from build123d import *

# Parameters (mm, degrees)
SKETCH_1_W      = 18
SKETCH_1_H      = 3
SKETCH_1_R      = 1.6
EXTRUDE_1_DEPTH = 1
FILLET_1_R      = 3
FILLET_2_R      = 1


with BuildPart() as part:
    # 草图1 → 凸台-拉伸1 (new body)
    with BuildSketch(Plane(origin=(0, 0, 0), x_dir=(1, 0, 0), z_dir=(0, 1, 0))):
        with BuildLine():
            Line((21, 20), (-21, 20))
            Line((-21, 20), (-34.150684932, 4.931506849))
            ThreePointArc((-34.150684932, 4.931506849), (-36, 0), (-34.150684932, -4.931506849))
            Line((-34.150684932, -4.931506849), (-21, -20))
            Line((-21, -20), (21, -20))
            Line((21, -20), (34.150684932, -4.931506849))
            ThreePointArc((34.150684932, -4.931506849), (36, 0), (34.150684932, 4.931506849))
            Line((34.150684932, 4.931506849), (21, 20))
        make_face()
        with Locations((-12, -15)):
            Rectangle(SKETCH_1_W, SKETCH_1_H, mode=Mode.SUBTRACT)
        with Locations((-12, -9)):
            Rectangle(SKETCH_1_W, SKETCH_1_H, mode=Mode.SUBTRACT)
        with Locations((-12, -3)):
            Rectangle(SKETCH_1_W, SKETCH_1_H, mode=Mode.SUBTRACT)
        with Locations((12, -15)):
            Rectangle(SKETCH_1_W, SKETCH_1_H, mode=Mode.SUBTRACT)
        with Locations((12, -9)):
            Rectangle(SKETCH_1_W, SKETCH_1_H, mode=Mode.SUBTRACT)
        with Locations((12, -3)):
            Rectangle(SKETCH_1_W, SKETCH_1_H, mode=Mode.SUBTRACT)
        with Locations((-12, 3)):
            Rectangle(SKETCH_1_W, SKETCH_1_H, mode=Mode.SUBTRACT)
        with Locations((-12, 9)):
            Rectangle(SKETCH_1_W, SKETCH_1_H, mode=Mode.SUBTRACT)
        with Locations((-12, 15)):
            Rectangle(SKETCH_1_W, SKETCH_1_H, mode=Mode.SUBTRACT)
        with Locations((12, 3)):
            Rectangle(SKETCH_1_W, SKETCH_1_H, mode=Mode.SUBTRACT)
        with Locations((12, 9)):
            Rectangle(SKETCH_1_W, SKETCH_1_H, mode=Mode.SUBTRACT)
        with Locations((12, 15)):
            Rectangle(SKETCH_1_W, SKETCH_1_H, mode=Mode.SUBTRACT)
        with Locations(Location((-28.5, 0, 0), (0, 0, 270))):
            Circle(SKETCH_1_R, mode=Mode.SUBTRACT)
        with Locations(Location((28.5, 0, 0), (0, 0, 270))):
            Circle(SKETCH_1_R, mode=Mode.SUBTRACT)
    extrude(amount=EXTRUDE_1_DEPTH)

    # 圆角1
    fillet_1_edges = [part.edges().sort_by_distance(p)[0] for p in [
        (21, 0.5, 20),
        (-21, 0.5, 20),
        (-21, 0.5, -20),
        (21, 0.5, -20),
    ]]
    fillet(fillet_1_edges, radius=FILLET_1_R)

    # 圆角2
    fillet_2_edges = [part.edges().sort_by_distance(p)[0] for p in [
        (-21, 0.5, 13.5),
        (-21, 0.5, 16.5),
        (-3, 0.5, 16.5),
        (-3, 0.5, 13.5),
        (21, 0.5, 16.5),
        (21, 0.5, 13.5),
        (3, 0.5, 13.5),
        (3, 0.5, 16.5),
        (21, 0.5, 10.5),
        (21, 0.5, 7.5),
        (3, 0.5, 7.5),
        (3, 0.5, 10.5),
        (21, 0.5, 4.5),
        (21, 0.5, 1.5),
        (3, 0.5, 1.5),
        (3, 0.5, 4.5),
        (21, 0.5, -1.5),
        (21, 0.5, -4.5),
        (3, 0.5, -4.5),
        (3, 0.5, -1.5),
        (21, 0.5, -7.5),
        (21, 0.5, -10.5),
        (3, 0.5, -10.5),
        (3, 0.5, -7.5),
        (21, 0.5, -13.5),
        (21, 0.5, -16.5),
        (3, 0.5, -16.5),
        (3, 0.5, -13.5),
        (-3, 0.5, 10.5),
        (-3, 0.5, 7.5),
        (-21, 0.5, 7.5),
        (-21, 0.5, 10.5),
        (-3, 0.5, 4.5),
        (-3, 0.5, 1.5),
        (-21, 0.5, 1.5),
        (-21, 0.5, 4.5),
        (-3, 0.5, -1.5),
        (-3, 0.5, -4.5),
        (-21, 0.5, -4.5),
        (-21, 0.5, -1.5),
        (-3, 0.5, -7.5),
        (-3, 0.5, -10.5),
        (-21, 0.5, -10.5),
        (-21, 0.5, -7.5),
        (-3, 0.5, -13.5),
        (-3, 0.5, -16.5),
        (-21, 0.5, -16.5),
        (-21, 0.5, -13.5),
    ]]
    fillet(fillet_2_edges, radius=FILLET_2_R)


solid = part.part
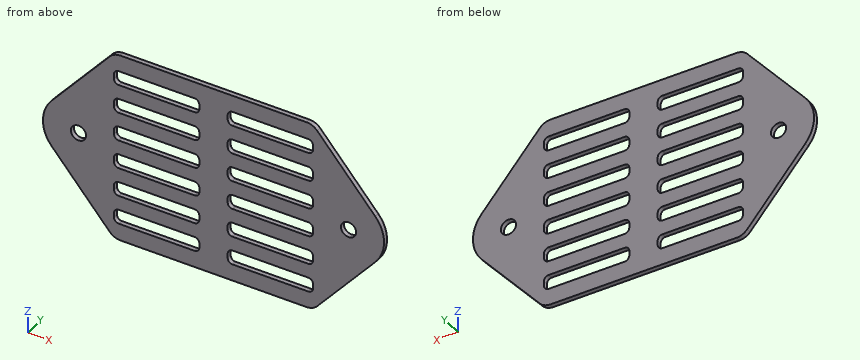
Verification items for the finished model (mm, model axes). Give positions to 0.01 mm unless a question says otherwise; leave off trailing zeros. Loops run counter-clockwise (first coordinate to the right, second up) from the corner with the lowest first, then second, coordinate; pieces in that order, holes last.
1) Sectioned sample at D-D, the plane y = 0.4. Count the separate pieces of the cut face and the enclosed holes in it, then the cut area to 3 significant figures.
2) Sectioned sample at C-C, the plane x = -28.5. Enter the section's corners in (y, z), then the cut area to 3 significant figures.
3) Thickness scan on line 1 along X through (y, z) = (0.9, -9.5); line 2 along X through (y, z) = (0.5, 14); line 3 along X through (y, z) = (0.25, 6.5). Record the ranges inside material, lowest first.
4) Depth check by flat-ended pin: pin 1 Ø0.5 at (y, z) = (0.5, 3) entering from -X. Enter the tip coordinate at first touch or a pass-through.
5) Sectioned sample at B-B, the plane z = 0. Enter the section's corners in (x, y).
6) Sectioned sample at A-A, the plane x = 5.5. Enter the section's corners in (y, z), then the cut area to 3 significant figures.
Answers:
1. separate pieces: 1
1. enclosed holes: 14
1. area: 1,710 mm2
2. outline: (0, -11.41) - (1, -11.41) - (1, -1.6) - (0, -1.6) - close; (0, 1.6) - (1, 1.6) - (1, 11.41) - (0, 11.41) - close
2. area: 19.6 mm2
3. line 1: x = -30.16 to -21, -3 to 3, 21 to 30.16
3. line 2: x = -26.24 to -20.87, -3.13 to 3.13, 20.87 to 26.24
3. line 3: x = -32.78 to 32.78
4. pin 1: stops at x = -35.48
5. outline: (-36, 0) - (-30.1, 0) - (-30.1, 1) - (-36, 1) - close; (-26.9, 0) - (26.9, 0) - (26.9, 1) - (-26.9, 1) - close; (30.1, 0) - (36, 0) - (36, 1) - (30.1, 1) - close
6. outline: (0, -20) - (1, -20) - (1, -16.5) - (0, -16.5) - close; (0, -13.5) - (1, -13.5) - (1, -10.5) - (0, -10.5) - close; (0, -7.5) - (1, -7.5) - (1, -4.5) - (0, -4.5) - close; (0, -1.5) - (1, -1.5) - (1, 1.5) - (0, 1.5) - close; (0, 4.5) - (1, 4.5) - (1, 7.5) - (0, 7.5) - close; (0, 10.5) - (1, 10.5) - (1, 13.5) - (0, 13.5) - close; (0, 16.5) - (1, 16.5) - (1, 20) - (0, 20) - close
6. area: 22.0 mm2
